from build123d import *

# Parameters (mm, degrees)
F1_W     = 5
F1_H     = 5
F1_R     = 1.6
F1_W_2   = 3
F1_H_2   = 7
F2_DEPTH = 5


with BuildPart() as f2:
    # F1 (on Top) → F2 (new body)
    with BuildSketch(Plane.XY):
        with BuildLine():
            ThreePointArc((30, 12), (29.1213203436, 14.1213203436), (27, 15))
            Line((27, 15), (-27, 15))
            ThreePointArc((-27, 15), (-29.1213203436, 14.1213203436), (-30, 12))
            Line((-30, 12), (-30, -35))
            Line((-30, -35), (-18, -35))
            Line((-18, -35), (-18, -32.5))
            Line((-18, -32.5), (-19.15, -32.5))
            Line((-19.15, -32.5), (-19.15, -30))
            Line((-19.15, -30), (-16.4, -30))
            Line((-16.4, -30), (-13.65, -30))
            Line((-13.65, -30), (-13.65, -32.5))
            Line((-13.65, -32.5), (-14.8, -32.5))
            Line((-14.8, -32.5), (-14.8, -35))
            Line((-14.8, -35), (-6, -35))
            Line((-6, -35), (-6, -25))
            ThreePointArc((-6, -25), (0, -19), (6, -25))
            Line((6, -25), (6, -35))
            Line((6, -35), (14.8, -35))
            Line((14.8, -35), (14.8, -32.5))
            Line((14.8, -32.5), (13.65, -32.5))
            Line((13.65, -32.5), (13.65, -30))
            Line((13.65, -30), (16.4, -30))
            Line((16.4, -30), (19.15, -30))
            Line((19.15, -30), (19.15, -32.5))
            Line((19.15, -32.5), (18, -32.5))
            Line((18, -32.5), (18, -35))
            Line((18, -35), (30, -35))
            Line((30, -35), (30, 12))
        make_face()
        with Locations((-24.5, -29.5)):
            Rectangle(F1_W, F1_H, mode=Mode.SUBTRACT)
        with Locations((-24.5, -23)):
            Circle(F1_R, mode=Mode.SUBTRACT)
        with Locations((-24.5, -16.5)):
            Rectangle(F1_W, F1_H, mode=Mode.SUBTRACT)
        with Locations((24.5, -29.5)):
            Rectangle(F1_W, F1_H, mode=Mode.SUBTRACT)
        with Locations((24.5, -23)):
            Circle(F1_R, mode=Mode.SUBTRACT)
        with Locations((24.5, -16.5)):
            Rectangle(F1_W, F1_H, mode=Mode.SUBTRACT)
        with Locations((-19.5, 0)):
            Rectangle(F1_W_2, F1_H_2, mode=Mode.SUBTRACT)
        with Locations((-5, -7.5)):
            Circle(F1_R, mode=Mode.SUBTRACT)
        with Locations((-5, 7.5)):
            Circle(F1_R, mode=Mode.SUBTRACT)
        with Locations((5, -7.5)):
            Circle(F1_R, mode=Mode.SUBTRACT)
        with Locations((19.5, 0)):
            Rectangle(F1_W_2, F1_H_2, mode=Mode.SUBTRACT)
        with Locations((5, 7.5)):
            Circle(F1_R, mode=Mode.SUBTRACT)
    extrude(amount=F2_DEPTH)


solid = f2.part
Design review of the part built by this model. Coordinates are the model's own, in mm. A direction names the side the tool comes from. Coordinates: 2 decimals unless noted, no trailing zeros. Loops run counter-clockwise (first coordinate to the right, second up) from the corner with the lowest first, then second, coordinate; pieces in that order, holes last.
Item 1: For faces 4 (the flat face through (18, -34, 2)), 5 (the flat face through (-10, -35, 2)), 6 (the flat face through (-21, 0, 2)), list the 3-axis set-ups (+Z, -Z, +X, -X, +Y, -Y) from which the entire face can be reached by the end or side of a thin tool; tool diameter is ignored.
Completed:
face 4: +Z, -Z, -Y
face 5: +Z, -Z, +X, -X, -Y
face 6: +Z, -Z
Item 2: Add section C-C (x = -20). Write out the cut boundary in (y, z), and give its area (3 significant figures).
Completed:
outline: (-35, 0) - (-3.5, 0) - (-3.5, 5) - (-35, 5) - close; (3.5, 0) - (15, 0) - (15, 5) - (3.5, 5) - close
area: 215 mm2
Item 3: Add section B-B (y = -7.5). Write out the cut boundary in (x, z).
Completed:
outline: (-30, 0) - (-6.6, 0) - (-6.6, 5) - (-30, 5) - close; (-3.4, 0) - (3.4, 0) - (3.4, 5) - (-3.4, 5) - close; (6.6, 0) - (30, 0) - (30, 5) - (6.6, 5) - close
Item 4: Add section A-A (x = 24.5). Write out the cut boundary in (y, z), and give its area (3 significant figures).
Completed:
outline: (-35, 0) - (-32, 0) - (-32, 5) - (-35, 5) - close; (-27, 0) - (-24.6, 0) - (-24.6, 5) - (-27, 5) - close; (-21.4, 0) - (-19, 0) - (-19, 5) - (-21.4, 5) - close; (-14, 0) - (15, 0) - (15, 5) - (-14, 5) - close
area: 184 mm2
Item 5: Add section D-D (y = -31). Write out the cut boundary in (x, z), and give its area (3 significant figures).
Completed:
outline: (-30, 0) - (-27, 0) - (-27, 5) - (-30, 5) - close; (-22, 0) - (-19.15, 0) - (-19.15, 5) - (-22, 5) - close; (-13.65, 0) - (-6, 0) - (-6, 5) - (-13.65, 5) - close; (6, 0) - (13.65, 0) - (13.65, 5) - (6, 5) - close; (19.15, 0) - (22, 0) - (22, 5) - (19.15, 5) - close; (27, 0) - (30, 0) - (30, 5) - (27, 5) - close
area: 135 mm2
Item 6: Wall thickness on L1, parallel to Y at x = 24.5, z = 3.1; L2, parallel to X at y = -18.5, z = 1; L3, parallel to X at y = -27.5, z = 3.75: over which ranges is each line inside the solid? List them lowest first.
Completed:
L1: y = -35 to -32, -27 to -24.6, -21.4 to -19, -14 to 15
L2: x = -30 to -27, -22 to 22, 27 to 30
L3: x = -30 to -27, -22 to -6, 6 to 22, 27 to 30
Item 7: Draft analysis for pull direction X (two halves, no side actions). For faces 1 (the flat face through (0, 15, 2)), 2 (the flat face through (-25, -27, 2)), 3 (the cylindrical face through (-29.1, 14.14, 2.46)), state which applies: pulls with the +X half, pulls with the -X half, needs draft (parallel to the pull), parting line crosses it, or undercut.
Completed:
face 1: needs draft
face 2: undercut
face 3: pulls with the -X half
Item 8: Clearance check with a flat-ended pin moving along its axis: pin 1 (4 mm diameter, centred on x = 12, y = -16, fed in from -Z). State where the tip first meets the part, or that it passes through.
Completed:
pin 1: stops at z = 0
